```python
from build123d import *

# Parameters (mm, degrees)
SKETCH1_W                    = 171.45
SKETCH1_H                    = 60
BOSS_EXTRUDE1_DEPTH          = 6.35
F_10_CLEARANCE_HOLE1_D       = 4.9784
SKETCH12_W                   = 14
SKETCH12_H                   = 7
CUT_EXTRUDE4_DEPTH           = 92.706409945
FILLET2_R                    = 2
FILLET2_OF_SKETCH_PATTERN1_R = 2
M5_CLEARANCE_HOLE2_D         = 5.3
M5_CLEARANCE_HOLE2_DEPTH     = 6
M5_CLEARANCE_HOLE3_D         = 5.3
M5_CLEARANCE_HOLE3_DEPTH     = 6


with BuildPart() as part:
    # Sketch1 → Boss-Extrude1 (new, symmetric)
    with BuildSketch(Plane.XY):
        Rectangle(SKETCH1_W, SKETCH1_H)
    extrude(amount=BOSS_EXTRUDE1_DEPTH, both=True)

    # #10 Clearance Hole1 (through all)
    with Locations(Plane.XY.offset(6.35)):
        with Locations((-80.9625, 17.625), (-80.9625, 3.3375), (-80.9625, -10.95), (-80.9625, -25.2375), (80.9625, 17.625), (80.9625, 3.3375), (80.9625, -10.95), (80.9625, -25.2375)):
            Hole(F_10_CLEARANCE_HOLE1_D / 2)

    # Sketch12 → Cut-Extrude4 (cut, through all)
    with BuildSketch(Plane.XY.offset(6.35)):
        with Locations((-57.15, 20.5)):
            Rectangle(SKETCH12_W, SKETCH12_H)
    cut_extrude4 = extrude(amount=-CUT_EXTRUDE4_DEPTH, mode=Mode.SUBTRACT)

    # Fillet2
    fillet2_edges = [part.edges().sort_by_distance(p)[0] for p in [
        (-50.15, 24, 0),
        (-50.15, 17, 0),
        (-64.15, 17, 0),
        (-64.15, 24, 0),
    ]]
    fillet(fillet2_edges, radius=FILLET2_R)

    # Sketch-Pattern1: Cut-Extrude4 at 7 more places
    with Locations((38.1, 0, 0), (76.2, 0, 0), (114.3, 0, 0), (114.3, -41, 0), (76.2, -41, 0), (0, -41, 0), (38.1, -41, 0)):
        add(cut_extrude4, mode=Mode.SUBTRACT)

    # Fillet2 of Sketch-Pattern1
    fillet2_of_sketch_pattern1_edges = [part.edges().sort_by_distance(p)[0] for p in [
        (-12.05, 24, 0),
        (-12.05, 17, 0),
        (-26.05, 17, 0),
        (-26.05, 24, 0),
        (26.05, 24, 0),
        (26.05, 17, 0),
        (12.05, 17, 0),
        (12.05, 24, 0),
        (64.15, 24, 0),
        (64.15, 17, 0),
        (50.15, 17, 0),
        (50.15, 24, 0),
        (64.15, -17, 0),
        (64.15, -24, 0),
        (50.15, -24, 0),
        (50.15, -17, 0),
        (26.05, -17, 0),
        (26.05, -24, 0),
        (12.05, -24, 0),
        (12.05, -17, 0),
        (-50.15, -17, 0),
        (-50.15, -24, 0),
        (-64.15, -24, 0),
        (-64.15, -17, 0),
        (-12.05, -17, 0),
        (-12.05, -24, 0),
        (-26.05, -24, 0),
        (-26.05, -17, 0),
    ]]
    fillet(fillet2_of_sketch_pattern1_edges, radius=FILLET2_OF_SKETCH_PATTERN1_R)

    # M5 Clearance Hole2
    with Locations(Plane(origin=(0, 30, 0), x_dir=(1, 0, 0), z_dir=(0, 1, 0))):
        with Locations((-57.15, 0), (-19.05, 0), (19.05, 0), (57.15, 0)):
            Hole(M5_CLEARANCE_HOLE2_D / 2, depth=M5_CLEARANCE_HOLE2_DEPTH)

    # M5 Clearance Hole3
    with Locations(Plane(origin=(0, -30, 0), x_dir=(-1, 0, 0), z_dir=(0, -1, 0))):
        with Locations((-57.15, 0), (-19.05, 0), (19.05, 0), (57.15, 0)):
            Hole(M5_CLEARANCE_HOLE3_D / 2, depth=M5_CLEARANCE_HOLE3_DEPTH)


solid = part.part
```
Can you work these out from the model? Positions are in its coordinate system, mm. A direction names the side the tool comes from. Give positions to 0.01 mm unless a question says otherwise; leave off trailing zeros. Write each loop counter-clockwise with the first axis right and the second up, starting at its lowest first coordinate (ties: lowest second). Pieces come first, ordered by that corner, then holes. Notation, with made-up numbers: (82, 36) - (114, 36) arc R27 ccw to (114, 73) - close; hole circle Ø9 at (-12.5, 85.25). An arc over 180 degrees is marked (long way). Write item = value, one per line. Start each with the question number.
1. Thinking about a two-plate mould opening in Z: for faces 4 (the face through (21.7, 27, -0.1)), 5 (the face through (78.663, 2.384, -0.089)), which applies, released by +Z, released by -Z, zero draft, split by the parting line, or undercut?
2. Please list where these lines run through material, in increasing order: line 1 (X direction, y = 22, z = 4) (3 decimals); line 2 (Y direction, x = -17.5, z = -5); line 3 (Z direction, x = 19, y = -28).
3. For pin 1 (4.5 mm diameter, centred on x = 80.96, y = 17.62, fed in from -Z), with a flat end and sliding along its axis, tell me the tip position at first contact or that it passes through.
4. Imagine slicing it at B-B (y = -10.95). Please give me the cut outline in (x, z) (3 decimals), and give its area (3 significant figures).
5. Imagine slicing it at A-A (x = 19.05). Please give me the cut outline in (y, z), and give its area (3 significant figures).
6. Imagine slicing it at C-C (z = 0). Count the separate pieces of the cut face and the enclosed holes in it, and give its area (3 significant figures).
7. On a 3-axis mill with a long thin cutter (end or side, diameter ignored), from which of +Z, -Z, +X, -X, +Y, -Y can I reach the whole of each face in a straight line? I mean faces 1 (the face through (-21.7, -27, -0.1)), 2 (the face through (-54.5, 27, -0.1)), 3 (the face through (64.15, 20, 0)). Say none if no direction works.
Worked answers:
q1.face_4 = undercut
q1.face_5 = zero draft
q2.line_1 = -85.725 to -64.15, -50.15 to -26.05, -12.05 to 12.05, 26.05 to 50.15, 64.15 to 85.725
q2.line_2 = -30 to -24, -17 to 17, 24 to 30
q2.line_3 = -6.35 to -2.65, 2.65 to 6.35
q3.pin_1 = through
q4.outline = (-85.725, -6.35) - (-83.452, -6.35) - (-83.452, 6.35) - (-85.725, 6.35) - close; (-78.473, -6.35) - (78.473, -6.35) - (78.473, 6.35) - (-78.473, 6.35) - close; (83.452, -6.35) - (85.725, -6.35) - (85.725, 6.35) - (83.452, 6.35) - close
q4.area = 2,050 mm2
q5.outline = (-30, -6.35) - (-24, -6.35) - (-24, -2.65) - (-30, -2.65) - close; (-30, 2.65) - (-24, 2.65) - (-24, 6.35) - (-30, 6.35) - close; (-17, -6.35) - (17, -6.35) - (17, 6.35) - (-17, 6.35) - close; (24, -6.35) - (30, -6.35) - (30, -2.65) - (24, -2.65) - close; (24, 2.65) - (30, 2.65) - (30, 6.35) - (24, 6.35) - close
q5.area = 521 mm2
q6.separate_pieces = 1
q6.enclosed_holes = 8
q6.area = 9,120 mm2
q7.face_1 = -Y
q7.face_2 = +Y
q7.face_3 = +Z, -Z
